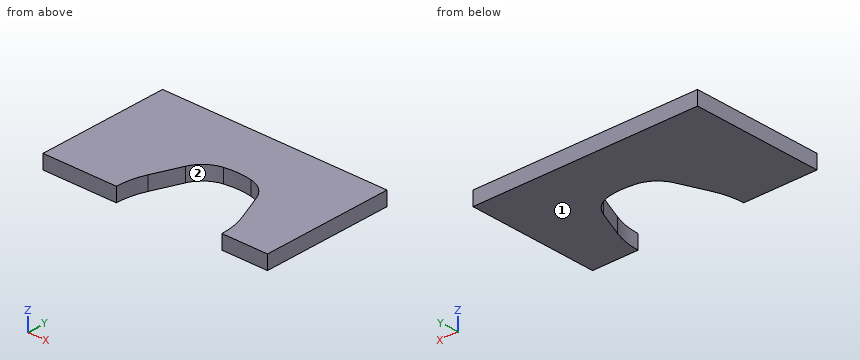
```python
from build123d import *

# Parameters (mm, degrees)
F1_DEPTH = 4.7752


with BuildPart() as f1:
    # F0 (on Top) → F1 (new body)
    with BuildSketch(Plane.XY):
        with BuildLine():
            Line((33.401, 44.323), (-42.799, 44.323))
            Line((-42.799, 44.323), (-42.799, 0))
            Line((-42.799, 0), (-17.907, 0))
            ThreePointArc((-17.907, 0), (-17.418946, 4.955294), (-15.97354, 9.720159))
            Line((-15.97354, 9.720159), (-12.015225, 19.276377))
            ThreePointArc((-12.015225, 19.276377), (-9.095689, 23.185245), (-4.664367, 25.226403))
            ThreePointArc((-4.664367, 25.226403), (0, 25.654), (4.664367, 25.226403))
            ThreePointArc((4.664367, 25.226403), (9.095689, 23.185245), (12.015225, 19.276377))
            Line((12.015225, 19.276377), (15.97354, 9.720159))
            ThreePointArc((15.97354, 9.720159), (17.418946, 4.955294), (17.907, 0))
            Line((17.907, 0), (33.401, 0))
            Line((33.401, 0), (33.401, 44.323))
        make_face()
    extrude(amount=F1_DEPTH)


solid = f1.part
```
The model under review builds one solid part; all positions refer to its coordinate system, in mm. Face numbers are marked on the shaded views. Round coordinates to 2 decimals unless told otherwise and drop trailing zeros. Loops run counter-clockwise (first coordinate to the right, second up) from the corner with the lowest first, then second, coordinate; pieces in that order, holes last. Notation, with made-up numbers: (5, -13.75) -> (9, -13.75) arc R18 ccw to (9, 18.25) -> close; hole circle Ø2 at (-16.5, 19.25). An arc over 180 degrees is marked (long way). Answer as a JSON object with one key per item and string values. Group by question number.
1) For line 1 (X direction, y = 2, z = 3.3); line 2 (X direction, y = 10, z = 1.05); line 3 (Y direction, x = 9.5, z = 0.95), list the stretches that pass through material, from the lowest coordinate up. Write a range as [from, to].
2) We need section C-C on y = 15. Write out the cut boundary in (x, z), then the cut area to 3 significant figures.
3) We need section A-A on y = 5. Write out the cut boundary in (x, z).
4) We need section B-B on z = 1.1. Write out the cut boundary in (x, y), then the cut area to 3 significant figures.
5) We need section D-D on x = 6. Write out the cut boundary in (y, z), then the cut area to 3 significant figures.
6) Mouldability with a two-part tool opening along X and no side actions: class the marked faces 1 and 2 as released by +X, released by -X, zero draft, split by the parting line, or undercut.
Result set:
{
 "1": {"line 1": "[-42.8, -17.83], [17.83, 33.4]", "line 2": "[-42.8, -15.86], [15.86, 33.4]", "line 3": "[22.84, 44.32]"},
 "2": {"outline": "(-42.8, 0) -> (-13.79, 0) -> (-13.79, 4.78) -> (-42.8, 4.78) -> close; (13.79, 0) -> (33.4, 0) -> (33.4, 4.78) -> (13.79, 4.78) -> close", "area": "232 mm²"},
 "3": {"outline": "(-42.8, 0) -> (-17.41, 0) -> (-17.41, 4.78) -> (-42.8, 4.78) -> close; (17.41, 0) -> (33.4, 0) -> (33.4, 4.78) -> (17.41, 4.78) -> close"},
 "4": {"outline": "(-42.8, 0) -> (-17.91, 0) arc R25.4 cw to (-15.97, 9.72) -> (-12.02, 19.28) arc R9.91 cw to (-4.66, 25.23) arc R25.65 cw to (4.66, 25.23) arc R9.91 cw to (12.02, 19.28) -> (15.97, 9.72) arc R25.4 cw to (17.91, 0) -> (33.4, 0) -> (33.4, 44.32) -> (-42.8, 44.32) -> close", "area": "2,660 mm²"},
 "5": {"outline": "(24.88, 0) -> (44.32, 0) -> (44.32, 4.78) -> (24.88, 4.78) -> close", "area": "92.8 mm²"},
 "6": {"face 1": "zero draft", "face 2": "undercut"}
}
